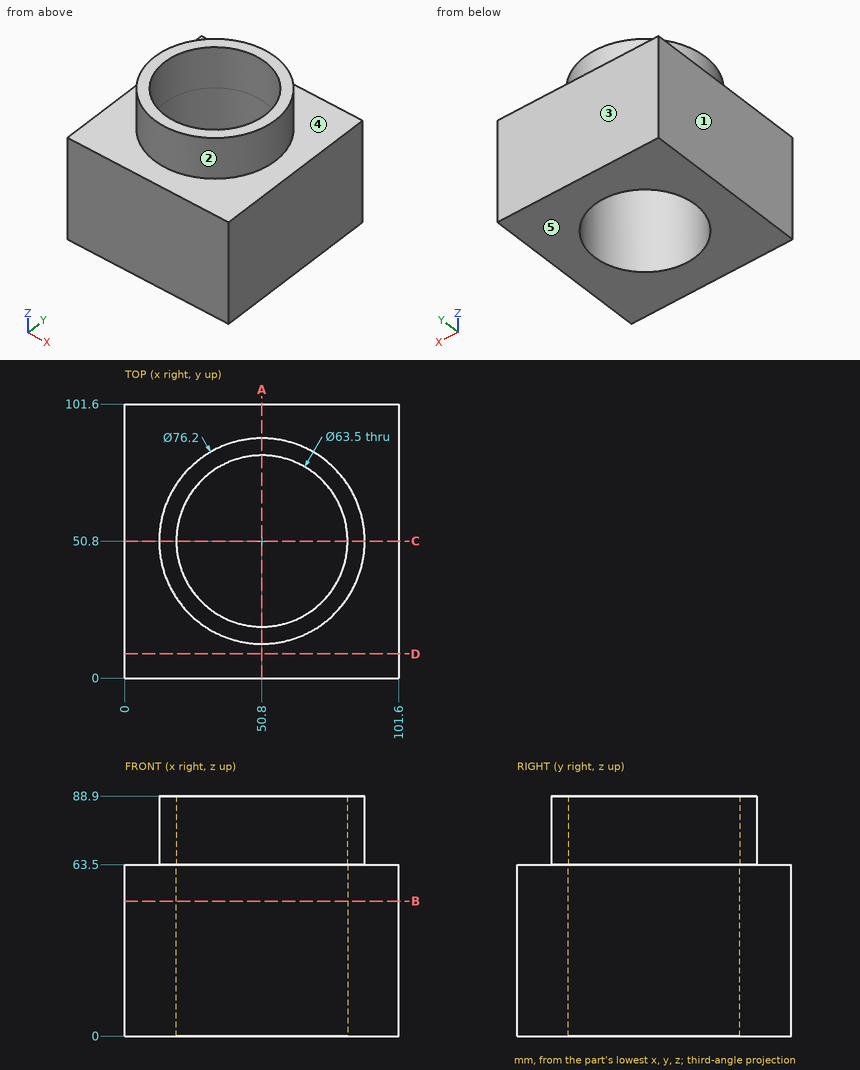
Design review of the part shown in the three views and the two pictorial views. Dimensions are in mm from the part's minimum x, y and z. A direction names the side the tool comes from. Give positions to 0.01 mm unless a question says otherwise; leave off trailing zeros. Write each loop counter-clockwise with the first axis right and the second up, starting at its lowest first coordinate (ties: lowest second). Pieces come first, ordered by that corner, then holes. Notation, with made-up numbers: M -36.5,-14.75 L -16.5,-14.75 A24 cw -16.5,23.25 Z; hole C -5.75,58 d7. An arc over 180 degrees is marked long. Answer as CSV lines item,"result".
1. Consider section A-A, the plane x = 50.8. Write out the cut boundary in (y, z).
Findings:
outline,"M 0,0 L 19.05,0 L 19.05,88.9 L 12.7,88.9 L 12.7,63.5 L 0,63.5 Z; M 82.55,0 L 101.6,0 L 101.6,63.5 L 88.9,63.5 L 88.9,88.9 L 82.55,88.9 Z"
2. Consider section B-B, the plane z = 50. Write out the cut boundary in (x, y), then the cut area to 3 significant figures.
Findings:
outline,"M 0,0 L 101.6,0 L 101.6,101.6 L 0,101.6 Z; hole C 50.8,50.8 d63.5"
area,"7,160 mm2"
3. Wall thickness on line 1 (Y direction, x = 50.8, z = 15); line 2 (X direction, y = 50, z = 27); line 3 (Z direction, x = 46, y = 89): over which ranges is each line inside the solid? List them lowest first.
Findings:
line 1,"y = 0 to 19.05, 82.55 to 101.6"
line 2,"x = 0 to 19.06, 82.54 to 101.6"
line 3,"z = 0 to 63.5"
4. Draft analysis for pull direction Y (two halves, no side actions). For the marked faces 1, 2 and 3, state which applies: +Y half, -Y half, draft (parallel to the pull), parting line (faces both ways), or undercut.
Findings:
face 1,"draft"
face 2,"parting line"
face 3,"+Y half"
5. For pin 1 (1.5 mm diameter, centred on x = 13, y = 18.5, fed in from +Z), flat-tipped, find the tip position at first contact; note if it passes through.
Findings:
pin 1,"stops at z = 63.5"
6. For the marked faces 4 and 5, list the 3-axis set-ups (+Z, -Z, +X, -X, +Y, -Y) from which the entire face can be reached by the end or side of a thin tool; tool diameter is ignored.
Findings:
face 4,"+Z"
face 5,"-Z, +X, -X, +Y, -Y"
7. Consider section D-D, the plane y = 9. Write out the cut boundary in (x, z), then the cut area to 3 significant figures.
Findings:
outline,"M 0,0 L 101.6,0 L 101.6,63.5 L 0,63.5 Z"
area,"6,450 mm2"
